Check sheet for the modelled part. Datum: model origin and axes. Units: mm. A direction names the side the tool comes from. Coordinates: 2 decimals unless noted, no trailing zeros. Loops run counter-clockwise (first coordinate to the right, second up) from the corner with the lowest first, then second, coordinate; pieces in that order, holes last. Notation, with made-up numbers: M 10,-35.5 L 39,-35.5 A14 cw 39,-24.5 Z; hole C 69,9.5 d8. An arc over 180 degrees is marked long. Write each question's results on one line, items separated by ' | '. Start each with the question number.
from build123d import *

# Parameters (mm, degrees)
BOSS_EXTRUDE1_DEPTH = 55
CUT_EXTRUDE1_REACH  = 193.293
SKETCH2_R           = 2.075
CUT_EXTRUDE2_REACH  = 196.404
SKETCH3_R           = 2.075
CUT_EXTRUDE3_DEPTH  = 3.2
CUT_EXTRUDE4_DEPTH  = 3.2
CUT_EXTRUDE5_REACH  = 193.293
SKETCH6_R           = 2.075
CUT_EXTRUDE6_DEPTH  = 3.2


with BuildPart() as part:
    # Sketch1 → Boss-Extrude1 (new body)
    with BuildSketch(Plane(origin=(0, 0, 0), x_dir=(0, 0, -1), z_dir=(1, 0, 0))):
        Polygon((0, -102), (0, -6), (10, -6), (10, 0), (0, 0), (-4, 0), (-4, -108), (148, -108), (148, -92), (142, -92), (142, -102), align=None)
    extrude(amount=BOSS_EXTRUDE1_DEPTH)

    # Sketch2 → Cut-Extrude1 (cut, up to next)
    with BuildSketch(Plane(origin=(0, 0, 0), x_dir=(1, 0, 0), z_dir=(0, 1, 0)), mode=Mode.PRIVATE) as cut_extrude1_sk1:
        with Locations(Location((10, 5, 0), (0, 0, 270))):
            Circle(SKETCH2_R)
    cut_extrude1_tool1 = extrude(cut_extrude1_sk1.sketch, amount=-CUT_EXTRUDE1_REACH, mode=Mode.PRIVATE) & part.part
    # Sketch2 → Cut-Extrude1 (cut, up to next)
    with BuildSketch(Plane(origin=(0, 0, 0), x_dir=(1, 0, 0), z_dir=(0, 1, 0)), mode=Mode.PRIVATE) as cut_extrude1_sk2:
        with Locations(Location((27.5, 5, 0), (0, 0, 270))):
            Circle(SKETCH2_R)
    cut_extrude1_tool2 = extrude(cut_extrude1_sk2.sketch, amount=-CUT_EXTRUDE1_REACH, mode=Mode.PRIVATE) & part.part
    # Sketch2 → Cut-Extrude1 (cut, up to next)
    with BuildSketch(Plane(origin=(0, 0, 0), x_dir=(1, 0, 0), z_dir=(0, 1, 0)), mode=Mode.PRIVATE) as cut_extrude1_sk3:
        with Locations(Location((45, 5, 0), (0, 0, 270))):
            Circle(SKETCH2_R)
    cut_extrude1_tool3 = extrude(cut_extrude1_sk3.sketch, amount=-CUT_EXTRUDE1_REACH, mode=Mode.PRIVATE) & part.part
    add(cut_extrude1_tool1.solids().sort_by_distance((10, 0, -5))[0], mode=Mode.SUBTRACT)
    add(cut_extrude1_tool2.solids().sort_by_distance((27.5, 0, -5))[0], mode=Mode.SUBTRACT)
    add(cut_extrude1_tool3.solids().sort_by_distance((45, 0, -5))[0], mode=Mode.SUBTRACT)

    # Sketch3 → Cut-Extrude2 (cut, up to next)
    with BuildSketch(Plane(origin=(0, 0, -148), x_dir=(-1, 0, 0), z_dir=(0, 0, -1)), mode=Mode.PRIVATE) as cut_extrude2_sk1:
        with Locations(Location((-45, -98, 0), (0, 0, 90))):
            Circle(SKETCH3_R)
    cut_extrude2_tool1 = extrude(cut_extrude2_sk1.sketch, amount=-CUT_EXTRUDE2_REACH, mode=Mode.PRIVATE) & part.part
    # Sketch3 → Cut-Extrude2 (cut, up to next)
    with BuildSketch(Plane(origin=(0, 0, -148), x_dir=(-1, 0, 0), z_dir=(0, 0, -1)), mode=Mode.PRIVATE) as cut_extrude2_sk2:
        with Locations(Location((-27.5, -98, 0), (0, 0, 90))):
            Circle(SKETCH3_R)
    cut_extrude2_tool2 = extrude(cut_extrude2_sk2.sketch, amount=-CUT_EXTRUDE2_REACH, mode=Mode.PRIVATE) & part.part
    # Sketch3 → Cut-Extrude2 (cut, up to next)
    with BuildSketch(Plane(origin=(0, 0, -148), x_dir=(-1, 0, 0), z_dir=(0, 0, -1)), mode=Mode.PRIVATE) as cut_extrude2_sk3:
        with Locations(Location((-10, -98, 0), (0, 0, 90))):
            Circle(SKETCH3_R)
    cut_extrude2_tool3 = extrude(cut_extrude2_sk3.sketch, amount=-CUT_EXTRUDE2_REACH, mode=Mode.PRIVATE) & part.part
    add(cut_extrude2_tool1.solids().sort_by_distance((45, -98, -148))[0], mode=Mode.SUBTRACT)
    add(cut_extrude2_tool2.solids().sort_by_distance((27.5, -98, -148))[0], mode=Mode.SUBTRACT)
    add(cut_extrude2_tool3.solids().sort_by_distance((10, -98, -148))[0], mode=Mode.SUBTRACT)

    # Sketch4 → Cut-Extrude3 (cut)
    with BuildSketch(Plane.XZ.offset(6)):
        Polygon((49.041451884, -5), (47.020725942, -1.5), (42.979274058, -1.5), (40.958548116, -5), (42.979274058, -8.5), (47.020725942, -8.5), align=None)
        Polygon((29.520725942, -8.5), (31.541451884, -5), (29.520725942, -1.5), (25.479274058, -1.5), (23.458548116, -5), (25.479274058, -8.5), align=None)
        Polygon((14.041451884, -5), (12.020725942, -1.5), (7.979274058, -1.5), (5.958548116, -5), (7.979274058, -8.5), (12.020725942, -8.5), align=None)
    extrude(amount=-CUT_EXTRUDE3_DEPTH, mode=Mode.SUBTRACT)

    # Sketch5 → Cut-Extrude4 (cut)
    with BuildSketch(Plane.XY.offset(-142)):
        Polygon((14.041451884, -98), (12.020725942, -94.5), (7.979274058, -94.5), (5.958548116, -98), (7.979274058, -101.5), (12.020725942, -101.5), align=None)
        Polygon((31.541451884, -98), (29.520725942, -94.5), (25.479274058, -94.5), (23.458548116, -98), (25.479274058, -101.5), (29.520725942, -101.5), align=None)
        Polygon((47.020725942, -101.5), (49.041451884, -98), (47.020725942, -94.5), (42.979274058, -94.5), (40.958548116, -98), (42.979274058, -101.5), align=None)
    extrude(amount=-CUT_EXTRUDE4_DEPTH, mode=Mode.SUBTRACT)

    # Sketch6 → Cut-Extrude5 (cut, up to next)
    with BuildSketch(Plane.XZ.offset(108), mode=Mode.PRIVATE) as cut_extrude5_sk1:
        with Locations(Location((46, -30.5, 0), (0, 0, 270))):
            Circle(SKETCH6_R)
    cut_extrude5_tool1 = extrude(cut_extrude5_sk1.sketch, amount=-CUT_EXTRUDE5_REACH, mode=Mode.PRIVATE) & part.part
    # Sketch6 → Cut-Extrude5 (cut, up to next)
    with BuildSketch(Plane.XZ.offset(108), mode=Mode.PRIVATE) as cut_extrude5_sk2:
        with Locations(Location((46, -70.5, 0), (0, 0, 270))):
            Circle(SKETCH6_R)
    cut_extrude5_tool2 = extrude(cut_extrude5_sk2.sketch, amount=-CUT_EXTRUDE5_REACH, mode=Mode.PRIVATE) & part.part
    # Sketch6 → Cut-Extrude5 (cut, up to next)
    with BuildSketch(Plane.XZ.offset(108), mode=Mode.PRIVATE) as cut_extrude5_sk3:
        with Locations(Location((9, -70.5, 0), (0, 0, 270))):
            Circle(SKETCH6_R)
    cut_extrude5_tool3 = extrude(cut_extrude5_sk3.sketch, amount=-CUT_EXTRUDE5_REACH, mode=Mode.PRIVATE) & part.part
    # Sketch6 → Cut-Extrude5 (cut, up to next)
    with BuildSketch(Plane.XZ.offset(108), mode=Mode.PRIVATE) as cut_extrude5_sk4:
        with Locations(Location((9, -30.5, 0), (0, 0, 270))):
            Circle(SKETCH6_R)
    cut_extrude5_tool4 = extrude(cut_extrude5_sk4.sketch, amount=-CUT_EXTRUDE5_REACH, mode=Mode.PRIVATE) & part.part
    add(cut_extrude5_tool1.solids().sort_by_distance((46, -108, -30.5))[0], mode=Mode.SUBTRACT)
    add(cut_extrude5_tool2.solids().sort_by_distance((46, -108, -70.5))[0], mode=Mode.SUBTRACT)
    add(cut_extrude5_tool3.solids().sort_by_distance((9, -108, -70.5))[0], mode=Mode.SUBTRACT)
    add(cut_extrude5_tool4.solids().sort_by_distance((9, -108, -30.5))[0], mode=Mode.SUBTRACT)

    # Sketch7 → Cut-Extrude6 (cut)
    with BuildSketch(Plane.XZ.offset(108)):
        Polygon((48.020725942, -27), (43.979274058, -27), (41.958548116, -30.5), (43.979274058, -34), (48.020725942, -34), (50.041451884, -30.5), align=None)
        Polygon((43.979274058, -74), (48.020725942, -74), (50.041451884, -70.5), (48.020725942, -67), (43.979274058, -67), (41.958548116, -70.5), align=None)
        Polygon((13.041451884, -70.5), (11.020725942, -74), (6.979274058, -74), (4.958548116, -70.5), (6.979274058, -67), (11.020725942, -67), align=None)
        Polygon((4.958548116, -30.5), (6.979274058, -27), (11.020725942, -27), (13.041451884, -30.5), (11.020725942, -34), (6.979274058, -34), align=None)
    extrude(amount=-CUT_EXTRUDE6_DEPTH, mode=Mode.SUBTRACT)


solid = part.part
1) Section check A-A (x = 38). Enter the section's corners in (y, z), then the cut area to 3 significant figures.
2) Release check for a two-part mould opening along Y. For faces 1 (the flat face through (7, -104.8, -72)), 2 (the flat face through (24.455, -99.726, -143.578)), 3 (the flat face through (12, -106.4, -68.7)) record: +Y half, -Y half, draft (parallel to the pull), parting line (faces both ways), or undercut.
3) Gauge pin test, flat ends, axial feed: P1, Ø2, axis at x = 25.5, y = -89.5, coming from the -Z side; P2, Ø3.5, axis at x = 10.5, z = -30.5, coming from the -Y side; P3, Ø3.5, axis at x = 27, z = -143.5, coming from the +Y side; P4, Ø3.5, axis at x = 46, z = -30.5, coming from the -Y side. Record the tip position at first contact, or that the pin passes through.
4) Section check D-D (z = -125). Enter the section's corners in (x, y), then the cut area to 3 significant figures.
5) Section check B-B (x = 27.5). Enter the section's corners in (y, z) (3 decimals), then the cut area to 3 significant figures.
6) Set-up check for faces 4 (the flat face through (49, -106.4, -32.3)), 5 (the cylindrical face through (7.74, -103.42, -28.85)), 6 (the flat face through (47, -100, -145.2)): record each of +Z, -Z, +X, -X, +Y, -Y from which the full face is reachable in a straight line by a thin tool's end or side.
7) Thickness scan on probe 1 along X at (y, z) = (-1.2, -5) (3 decimals); probe 2 along X at (y, z) = (-103, -30); probe 3 along Y at (x, z) = (47.5, -5). Record the ranges inside material, lowest first.
8) Section check C-C (y = -27). Enter the section's corners in (x, z), then the cut area to 3 significant figures.
Return value:
1) outline: M -108,-148 L -92,-148 L -92,-142 L -102,-142 L -102,0 L -6,0 L -6,-10 L 0,-10 L 0,4 L -108,4 Z | area: 1,440 mm2
2) face 1: -Y half | face 2: undercut | face 3: draft
3) P1: stops at z = 0 | P2: stops at y = -104.8 | P3: stops at y = -92 | P4: passes through
4) outline: M 0,-108 L 55,-108 L 55,-102 L 0,-102 Z | area: 330 mm2
5) outline: M -108,-148 L -100.075,-148 L -100.075,-145.2 L -101.5,-145.2 L -101.5,-142 L -102,-142 L -102,0 L -6,0 L -6,-1.5 L -2.8,-1.5 L -2.8,-2.925 L 0,-2.925 L 0,4 L -108,4 Z; M -95.925,-148 L -92,-148 L -92,-142 L -94.5,-142 L -94.5,-145.2 L -95.925,-145.2 Z; M -6,-10 L 0,-10 L 0,-7.075 L -2.8,-7.075 L -2.8,-8.5 L -6,-8.5 Z | area: 1,370 mm2
6) face 4: -Y | face 5: +Y, -Y | face 6: none
7) probe 1: x = 0 to 7.925, 12.075 to 25.425, 29.575 to 42.925, 47.075 to 55 | probe 2: x = 0 to 6.99, 11.01 to 43.99, 48.01 to 55 | probe 3: y = -108 to -102, -2.8 to 0
8) outline: M 0,0 L 55,0 L 55,4 L 0,4 Z | area: 220 mm2
